```python
from build123d import *

# Parameters (mm, degrees)
SKETCH_1_R          = 11
SKETCH_1_R_2        = 1.5
EXTRUDE_1_DEPTH     = 22
CUT_EXTRUDE_START   = -1.5
SKETCH_2_R          = 12.5
SKETCH_2_R_2        = 10
CUT_EXTRUDE_1_DEPTH = 19
SKETCH_3_R          = 1
CUT_EXTRUDE_2_DEPTH = 18
CHAMFER_1_SIZE      = 0.5
CHAMFER_2_SIZE      = 0.5
SKETCH_4_R          = 8.5
CUT_EXTRUDE_3_DEPTH = 10


with BuildPart() as part:
    # Эскиз1 → Бобышка-Вытянуть1 (new body)
    with BuildSketch(Plane(origin=(0, 0, 0), x_dir=(1, 0, 0), z_dir=(0, 1, 0))):
        with Locations(Location((0, 0, 0), (0, 0, 270))):
            Circle(SKETCH_1_R)
        with Locations(Location((0, 0, 0), (0, 0, 270))):
            Circle(SKETCH_1_R_2, mode=Mode.SUBTRACT)
    extrude(amount=EXTRUDE_1_DEPTH)

    # Эскиз2 → Вырез-Вытянуть1 (cut)
    with BuildSketch(Plane(origin=(0, 22, 0), x_dir=(1, 0, 0), z_dir=(0, 1, 0)).offset(CUT_EXTRUDE_START)):
        Circle(SKETCH_2_R)
        with Locations(Location((0, 0, 0), (0, 0, 270))):
            Circle(SKETCH_2_R_2, mode=Mode.SUBTRACT)
    extrude(amount=-CUT_EXTRUDE_1_DEPTH, mode=Mode.SUBTRACT)

    # Эскиз3 → Вырез-Вытянуть2 (cut)
    with BuildSketch(Plane(origin=(0, 0, 0), x_dir=(0, 0, -1), z_dir=(1, 0, 0))):
        with Locations((0, 4.529870325)):
            Circle(SKETCH_3_R)
    extrude(amount=-CUT_EXTRUDE_2_DEPTH, mode=Mode.SUBTRACT)

    # Фаска1
    chamfer_1_edges = [part.edges().sort_by_distance(p)[0] for p in [
        (0, 0, -11),
    ]]
    chamfer(chamfer_1_edges, length=CHAMFER_1_SIZE)

    # Фаска2
    chamfer_2_edges = [part.edges().sort_by_distance(p)[0] for p in [
        (0, 22, -11),
    ]]
    chamfer(chamfer_2_edges, length=CHAMFER_2_SIZE)

    # Эскиз4 → Вырез-Вытянуть3 (cut)
    with BuildSketch(Plane(origin=(0, 22, 0), x_dir=(1, 0, 0), z_dir=(0, 1, 0))):
        with Locations(Location((0, 0, 0), (0, 0, 270))):
            Circle(SKETCH_4_R)
    extrude(amount=-CUT_EXTRUDE_3_DEPTH, mode=Mode.SUBTRACT)


solid = part.part
```
Part model, mm, in its own coordinate system. A direction names the side the tool comes from. Round coordinates to 2 decimals unless told otherwise and drop trailing zeros. Loops run counter-clockwise (first coordinate to the right, second up) from the corner with the lowest first, then second, coordinate; pieces in that order, holes last. Notation, with made-up numbers: (54, 23.5) -> (95, 23.5) arc R13 ccw to (95, 42.5) -> close; hole circle Ø2 at (40, -19.5). An arc over 180 degrees is marked (long way). Use one line per item in the form item = value. Start each with the question number.
Item 1: Drill centre lines: line 1 along Y through (x, z) = (-6.5, 0); line 2 along X through (y, z) = (16, 0); line 3 along Z through (x, y) = (-6.5, 17). Where is each one in solid material? Low to high.
Item 2: Two-plate mould, pull along Y, no slides. Class faces 1 (the flat face through (-2, 12, 0)), 2 (the flat face through (2, 1.5, 10)), 3 (the cylindrical face through (8.428, 17.07, -1.107)): released by +Y, released by -Y, zero draft, split by the parting line, or undercut.
Item 3: Tool access for faces 4 (the cylindrical face through (-5.498, 3.554, 0.217)), 5 (the flat face through (0, 22, 9)), 6 (the flat face through (2, 20.5, 10)): list every direction of +Z, -Z, +X, -X, +Y, -Y with a clear straight run to the whole face (end or side of a thin tool).
Item 4: Drop flat-ended pins along their axis: pin 1 Ø1.6 at (y, z) = (4.53, 0) entering from +X; pin 2 Ø10 at (y, z) = (11.5, -8) entering from -X; pin 3 Ø8.5 at (x, z) = (-4, -0.5) entering from +Y. Give the stop position or say it passes through.
Item 5: Band-saw the part on C-C (y = 6). List the corners of the cut face in (x, z), plus the area to 3 significant figures.
Item 6: Band-saw the part on A-A (x = 0). List the corners of the cut face in (y, z), plus the area to 4 significant figures.
Item 7: Band-saw the part on B-B (z = 0). List the corners of the cut face in (x, y), plus the area to 4 significant figures.
Item 8: Band-saw the part on D-D (y = 13.5). List the corners of the cut face in (x, z).
Data:
q1.line_1 = 0 to 3.53, 5.53 to 12
q1.line_2 = -10 to -8.5, 8.5 to 10
q1.line_3 = -7.6 to -5.48, 5.48 to 7.6
q2.face_1 = released by +Y
q2.face_2 = undercut
q2.face_3 = zero draft
q3.face_4 = -X
q3.face_5 = +Z, -Z, +X, -X, +Y
q3.face_6 = none
q4.pin_1 = 10
q4.pin_2 = -9.54
q4.pin_3 = 12
q5.outline = circle Ø20 at (0, 0); hole circle Ø3 at (0, 0)
q5.area = 307 mm^2
q6.outline = (0, -10.5) -> (0.5, -11) -> (1.5, -11) -> (1.5, -10) -> (20.5, -10) -> (20.5, -11) -> (21.5, -11) -> (22, -10.5) -> (22, -8.5) -> (12, -8.5) -> (12, -1.5) -> (0, -1.5) -> close; (0, 1.5) -> (12, 1.5) -> (12, 8.5) -> (22, 8.5) -> (22, 10.5) -> (21.5, 11) -> (20.5, 11) -> (20.5, 10) -> (1.5, 10) -> (1.5, 11) -> (0.5, 11) -> (0, 10.5) -> close
q6.area = 239.5 mm^2
q7.outline = (-11, 0.5) -> (-10.5, 0) -> (-1.5, 0) -> (-1.5, 3.53) -> (-10, 3.53) -> (-10, 1.5) -> (-11, 1.5) -> close; (-11, 20.5) -> (-10, 20.5) -> (-10, 5.53) -> (-1.5, 5.53) -> (-1.5, 12) -> (-8.5, 12) -> (-8.5, 22) -> (-10.5, 22) -> (-11, 21.5) -> close; (1.5, 0) -> (10.5, 0) -> (11, 0.5) -> (11, 1.5) -> (10, 1.5) -> (10, 20.5) -> (11, 20.5) -> (11, 21.5) -> (10.5, 22) -> (8.5, 22) -> (8.5, 12) -> (1.5, 12) -> close
q7.area = 222.5 mm^2
q8.outline = circle Ø20 at (0, 0); hole circle Ø17 at (0, 0)
